```python
from build123d import *

# Parameters (mm, degrees)
SKETCH1_R          = 43.5
SKETCH1_R_2        = 32.5
BODY_DEPTH         = 4
SKETCH2_R          = 2.5
BOLT_HOLE_DEPTH    = 62.648195432
BOLT_PATTERN_COUNT = 12


with BuildPart() as part:
    # Sketch1 → Body (new body)
    with BuildSketch(Plane.XY):
        Circle(SKETCH1_R)
        Circle(SKETCH1_R_2, mode=Mode.SUBTRACT)
    extrude(amount=BODY_DEPTH)

    # Sketch2 → Bolt Hole (cut, through all)
    with BuildSketch(Plane.XY.offset(4)):
        with Locations((0, 38)):
            Circle(SKETCH2_R)
    bolt_hole = extrude(amount=-BOLT_HOLE_DEPTH, mode=Mode.SUBTRACT)

    # Bolt Pattern: Bolt Hole ×12 about axis
    bolt_pattern_axis = Axis((0, 0, 0), (0, 0, 1))
    for i in range(1, BOLT_PATTERN_COUNT):
        add(bolt_hole.rotate(bolt_pattern_axis, i * 360 / BOLT_PATTERN_COUNT), mode=Mode.SUBTRACT)


solid = part.part
```
Here's how the part is built. I have some questions about the finished solid (model axes, mm). Round coordinates to 2 decimals unless told otherwise and drop trailing zeros. Write each loop counter-clockwise with the first axis right and the second up, starting at its lowest first coordinate (ties: lowest second). Pieces come first, ordered by that corner, then holes.
Q1. If we section it at A-A on x = 0: Write out the boundary of the cut face in (y, z).
Q2. If we section it at B-B on y = 11.5: Write out the boundary of the cut face in (x, z).
Q3. If we section it at D-D on x = -37: Write out the boundary of the cut face in (y, z), plus the area to 3 significant figures.
Q4. Please list where these lines run through material, in increasing order: probe 1 along Y at (x, z) = (0, 1.4); probe 2 along Y at (x, z) = (20, 1); probe 3 along Y at (x, z) = (35, 1.5).
Q5. If we section it at C-C on z = 1: Give the number of separate pieces and of enclosed holes in the cut face, plus the area to 3 significant figures.
Q6. Will these pins go through, and if not, where does the flat tip stop? P1, Ø6.5, axis at x = 32.91, y = 19, coming from the -Z side; P2, Ø1, axis at x = -25.5, z = 2.5, coming from the +Y side; P3, Ø4.5, axis at x = -38, y = 0, coming from the +Z side; P4, Ø1, axis at y = -34.5, z = 3, coming from the +X side.
Q7. If we mould it in two halves opening along Y, with no side actions, what happens to faces 1 (the cylindrical face through (18.249, -30.524, 2.028)), 2 (the flat face through (-16, 29, 4)), 3 (the cylindrical face through (-5.66, 43.13, 1.97))? For each: +Y half, -Y half, draft (parallel to the pull), parting line (faces both ways), or undercut.
Answer below:
1. outline: (-43.5, 0) - (-40.5, 0) - (-40.5, 4) - (-43.5, 4) - close; (-35.5, 0) - (-32.5, 0) - (-32.5, 4) - (-35.5, 4) - close; (32.5, 0) - (35.5, 0) - (35.5, 4) - (32.5, 4) - close; (40.5, 0) - (43.5, 0) - (43.5, 4) - (40.5, 4) - close
2. outline: (-41.95, 0) - (-30.4, 0) - (-30.4, 4) - (-41.95, 4) - close; (30.4, 0) - (41.95, 0) - (41.95, 4) - (30.4, 4) - close
3. outline: (-22.87, 0) - (-2.29, 0) - (-2.29, 4) - (-22.87, 4) - close; (2.29, 0) - (22.87, 0) - (22.87, 4) - (2.29, 4) - close
3. area: 165 mm2
4. probe 1: y = -43.5 to -40.5, -35.5 to -32.5, 32.5 to 35.5, 40.5 to 43.5
4. probe 2: y = -38.63 to -35.2, -30.62 to -25.62, 25.62 to 30.62, 35.2 to 38.63
4. probe 3: y = -25.83 to -20.37, -17.63 to 17.63, 20.37 to 25.83
5. separate pieces: 1
5. enclosed holes: 13
5. area: 2,390 mm2
6. P1: stops at z = 0
6. P2: stops at y = 35.6
6. P3: passes through
6. P4: stops at x = 27.13
7. face 1: undercut
7. face 2: draft
7. face 3: parting line
